CAD build for the part. Positions are in the model's coordinates, mm. Face numbers are marked on the shaded views. A direction names the side the tool comes from. Give positions to 0.01 mm unless a question says otherwise; leave off trailing zeros. Order: outer loops, then holes, each group sorted by start corner. A loop starts at its lowest first (then second) coordinate and runs counter-clockwise, first axis right, second up.
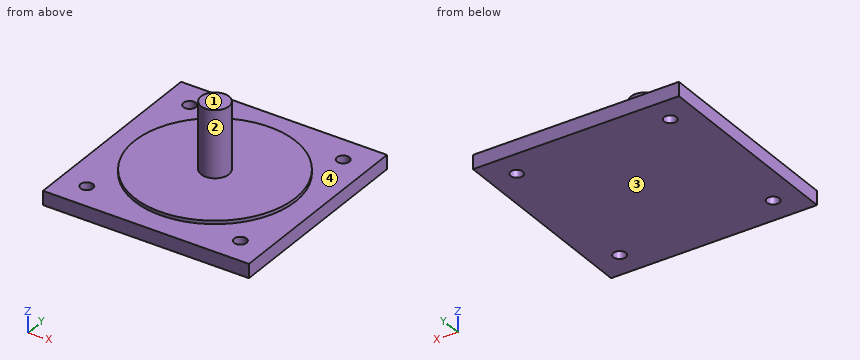
from build123d import *

# Parameters (mm, degrees)
F0_W     = 93.345
F0_H     = 93.345
F1_DEPTH = 6.35
F2_R     = 36.5125
F3_DEPTH = 1.524
F4_R     = 6.35
F5_DEPTH = 31.75
F6_R     = 2.8321
F7_DEPTH = 6.35


with BuildPart() as f1:
    # F0 (on Top) → F1 (new body)
    with BuildSketch(Plane.XY):
        Rectangle(F0_W, F0_H)
    extrude(amount=F1_DEPTH)

    # F2 (on face) → F3 (join)
    with BuildSketch(Plane.XY.offset(6.35)):
        Circle(F2_R)
    extrude(amount=F3_DEPTH)

    # F4 (on face) → F5 (join)
    with BuildSketch(Plane.XY.offset(6.35)):
        Circle(F4_R)
    extrude(amount=F5_DEPTH)

    # F6 (on face) → F7 (cut, through all)
    with BuildSketch(Plane.XY.offset(6.35)):
        with Locations((-34.798, 34.798)):
            Circle(F6_R)
        with Locations((34.798, 34.798)):
            Circle(F6_R)
        with Locations((34.798, -34.798)):
            Circle(F6_R)
        with Locations((-34.798, -34.798)):
            Circle(F6_R)
    extrude(amount=-F7_DEPTH, mode=Mode.SUBTRACT)


solid = f1.part
1. 3-axis set-ups, long thin cutter, end or side, ignore diameter. For the marked faces 3 and 4: which of +Z, -Z, +X, -X, +Y, -Y reach the whole face in a straight line?
2. Saw through at D-D on y = 19. Give the cut face in (x, z).
3. Mould opens along X. For the marked faces 1 and 2 say: released by +X, released by -X, zero draft, split by the parting line, or undercut.
4. Saw through at A-A on x = 0. Give the cut face in (y, z), plus the area to 3 significant figures.
5. Pin check, flat tips, straight feed: P1, Ø7.5, axis at x = 34.798, y = -34.798, coming from the -Z side; P2, Ø10, axis at y = -1.5, z = 13, coming from the +X side; P3, Ø8, axis at x = -11.5, y = -16, coming from the +Z side; P4, Ø7.5, axis at x = 34.798, y = 34.798, coming from the +Z side. Stop position of each tip, or through.
6. Saw through at C-C on z = 26.5. Give the cut face in (x, y).
7. Wall check: line 1 (Z direction, x = -37, y = -10); line 2 (Z direction, x = -15, y = -23); line 3 (X direction, y = -0.5, z = 10.5). Give the ranges that are in metal, low to high.
Reported:
1. face 3: -Z, +X, -X, +Y, -Y
1. face 4: +Z
2. outline: (-46.67, 0) - (46.67, 0) - (46.67, 6.35) - (31.18, 6.35) - (31.18, 7.87) - (-31.18, 7.87) - (-31.18, 6.35) - (-46.67, 6.35) - close
3. face 1: zero draft
3. face 2: split by the parting line
4. outline: (-46.67, 0) - (46.67, 0) - (46.67, 6.35) - (36.51, 6.35) - (36.51, 7.87) - (6.35, 7.87) - (6.35, 38.1) - (-6.35, 38.1) - (-6.35, 7.87) - (-36.51, 7.87) - (-36.51, 6.35) - (-46.67, 6.35) - close
4. area: 1,090 mm2
5. P1: stops at z = 0
5. P2: stops at x = 6.35
5. P3: stops at z = 7.87
5. P4: stops at z = 6.35
6. outline: circle Ø12.7 at (0, 0)
7. line 1: z = 0 to 6.35
7. line 2: z = 0 to 7.87
7. line 3: x = -6.33 to 6.33
